Job drawing, mm, ordinate dimensions from the low corner. One solid piece. A direction names the side the tool comes from. Give positions to 0.01 mm unless a question says otherwise; leave off trailing zeros. Write each loop counter-clockwise with the first axis right and the second up, starting at its lowest first coordinate (ties: lowest second). Pieces come first, ordered by that corner, then holes. Notation, with made-up numbers: M 28.25,-25 L 43.25,-25 A17 ccw 43.25,7 Z; hole C -26,51 d11. An arc over 180 degrees is marked long. Use CSV: the item, a comma, the result in double quotes. Start each with the question number.
Item 1: Drill centre lines: line 1 (Y direction, x = 65, z = 8); line 2 (Y direction, x = 112.5, z = 9); line 3 (Y direction, x = 70, z = 14). Where is each one in solid material? Low to high. Write a range as [from, to].
Item 2: Cut at A-A (x = 65). List the corners of the cut face in (y, z), then the cut area to 3 significant figures.
Item 3: Mould opens along Y. For the marked faces 1, 2 and 3 say: released by +Y, released by -Y, zero draft, split by the parting line, or undercut.
Item 4: Cut at D-D (x = 15). List the corners of the cut face in (y, z).
Item 5: Pin check, flat tip, straight feed: pin 1 (1.5 mm diameter, centred on x = 109.5, z = 11.5, fed in from -Y). Stop position of the tip, or through.
Item 6: Which spindle directions (+Z, -Z, +X, -X, +Y, -Y) get a long thin tool onto all of the face, cutting with end or side? Do the marked faces 4 and 5. Say none if no direction does.
Item 7: Cut at B-B (y = 145). List the corners of the cut face in (x, z).
Item 8: Cut at C-C (z = 21.75). List the corners of the cut face in (x, y) (1 decimal).
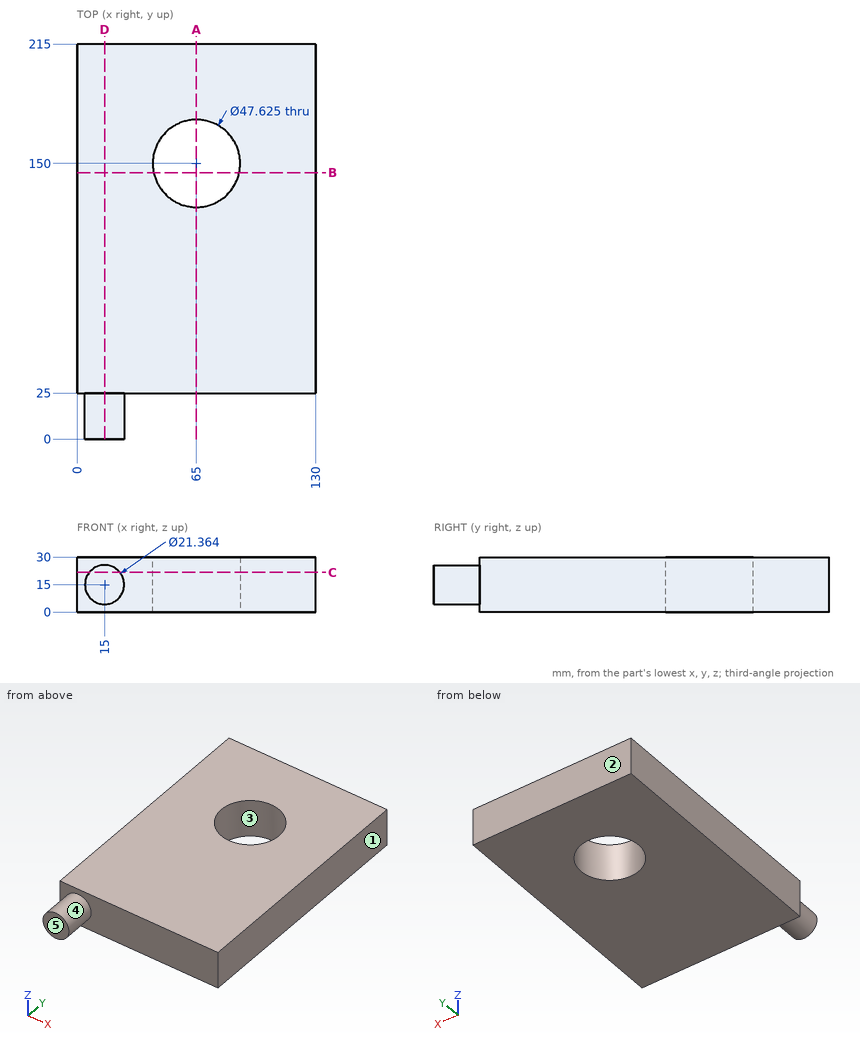
Worked answers:
1,line 1,"y = [25, 126.19], [173.81, 215]"
1,line 2,"y = [25, 215]"
1,line 3,"y = [25, 126.72], [173.28, 215]"
2,outline,"M 25,0 L 126.19,0 L 126.19,30 L 25,30 Z; M 173.81,0 L 215,0 L 215,30 L 173.81,30 Z"
2,area,"4,270 mm^2"
3,face 1,"zero draft"
3,face 2,"released by +Y"
3,face 3,"undercut"
4,outline,"M 0,4.32 L 25,4.32 L 25,0 L 215,0 L 215,30 L 25,30 L 25,25.68 L 0,25.68 Z"
5,pin 1,"stops at y = 25"
6,face 4,"-Y"
6,face 5,"+Z, -Z, +X, -X, -Y"
7,outline,"M 0,0 L 41.72,0 L 41.72,30 L 0,30 Z; M 88.28,0 L 130,0 L 130,30 L 88.28,30 Z"
8,outline,"M 0,25 L 6.7,25 L 6.7,0 L 23.3,0 L 23.3,25 L 130,25 L 130,215 L 0,215 Z; hole C 65,150 d47.6"
